from build123d import *

# Parameters (mm, degrees)
F0_R        = 8.4621636151
F0_R_2      = 8.6410874337
F1_DEPTH    = 50
F4_T1_DEPTH = 125
F4_T3_DEPTH = 75.1791274175
F4_T8_DEPTH = 127.0995380357


# Not quite as in the source:
# - a fillet or chamfer that OpenCascade refuses, or shapes differently, is made with other operations: its cross-section is extruded or revolved along the edge and cut away or added
# - a feature of the source that left no trace in its solid (it failed there, or was rolled back) is left out


with BuildPart() as f1:
    # F0 (on Front) → F1 (new body)
    with BuildSketch(Plane.XZ):
        with BuildLine():
            Line((-12.9085844383, 52.6810027659), (-60.1237900555, 52.6810027659))
            Line((-60.1237900555, 52.6810027659), (-60.1237900555, 27.209569862))
            ThreePointArc((-60.1237900555, 27.209569862), (-40.7058920955, 7.7916719019), (-60.1237900555, -11.6262260581))
            Line((-60.1237900555, -11.6262260581), (-60.1237900555, -42.4471646547))
            Line((-60.1237900555, -42.4471646547), (-12.2108235955, -42.4471646547))
            Line((-12.2108235955, -42.4471646547), (-12.2108235955, -22.2120806575))
            Line((-12.2108235955, -22.2120806575), (11.7456596345, -22.2120806575))
            Line((11.7456596345, -22.2120806575), (11.7456596345, -42.4471646547))
            Line((11.7456596345, -42.4471646547), (60.588978231, -42.4471646547))
            Line((60.588978231, -42.4471646547), (60.588978231, 0))
            Line((60.588978231, 0), (13.5322010265, 0))
            ThreePointArc((13.5322010265, 0), (4.0349011674, 7.5009376742), (13.5322010265, 15.0018753484))
            Line((13.5322010265, 15.0018753484), (60.588978231, 15.0018753484))
            Line((60.588978231, 15.0018753484), (60.588978231, 52.6810027659))
            Line((60.588978231, 52.6810027659), (8.4894401953, 52.6810027659))
            Line((8.4894401953, 52.6810027659), (8.4894401953, 30.5852182209))
            Line((8.4894401953, 30.5852182209), (-12.9085844383, 30.5852182209))
            Line((-12.9085844383, 30.5852182209), (-12.9085844383, 52.6810027659))
        make_face()
        with Locations((40.4487065971, -18.1611850858)):
            Circle(F0_R, mode=Mode.SUBTRACT)
        with Locations((37.1295772493, 35.4981198907)):
            Circle(F0_R_2, mode=Mode.SUBTRACT)
    extrude(amount=F1_DEPTH)

    # F4: fillet of radius 15 on 3 edges, made by hand

    # F4_s2 → F4_t1 (cut)
    with BuildSketch(Plane.XZ.offset(-37.5)):
        with BuildLine():
            ThreePointArc((45.588978231, -42.4471646547), (56.1955799488, -38.0537663725), (60.588978231, -27.4471646547))
            Line((60.588978231, -27.4471646547), (60.588978231, -42.4471646547))
            Line((60.588978231, -42.4471646547), (45.588978231, -42.4471646547))
        make_face()
    extrude(amount=F4_T1_DEPTH, mode=Mode.SUBTRACT)

    # F4_s4 → F4_t3 (cut)
    with BuildSketch(Plane.XY.offset(15.0018753484)):
        with BuildLine():
            ThreePointArc((60.588978231, -15), (56.1955799488, -4.3933982822), (45.588978231, 0))
            Line((45.588978231, 0), (60.588978231, 0))
            Line((60.588978231, 0), (60.588978231, -15))
        make_face()
    extrude(amount=F4_T3_DEPTH, mode=Mode.SUBTRACT)


with BuildPart() as f4_tool6:
    # F4_s7 → F4_t8 (new body)
    with BuildSketch(Plane.YZ.offset(98.088978231)):
        with BuildLine():
            ThreePointArc((-35, 52.6810027659), (-45.6066017178, 48.2876044837), (-50, 37.6810027659))
            Line((-50, 37.6810027659), (-50, 52.6810027659))
            Line((-50, 52.6810027659), (-35, 52.6810027659))
        make_face()
    extrude(amount=-F4_T8_DEPTH)

    split(bisect_by=Plane.YZ.offset(-12.9085844383), keep=Keep.TOP)


with BuildPart() as f1_1:
    add(f1.part)

    # F4_t5: cut F4_tool6
    add(f4_tool6.part, mode=Mode.SUBTRACT)


solid = f1_1.part
Model file for the job. Use its own axes, mm. A direction names the side the tool comes from. Round coordinates to 2 decimals unless told otherwise and drop trailing zeros. Loops run counter-clockwise (first coordinate to the right, second up) from the corner with the lowest first, then second, coordinate; pieces in that order, holes last.
1. Band-saw the part on D-D, the plane z = -24.5. List the corners of the cut face in (x, y).
Check values:
outline: (-60.12, -50) - (-12.21, -50) - (-12.21, 0) - (-60.12, 0) - close; (11.75, -50) - (34.84, -50) - (34.84, 0) - (11.75, 0) - close; (46.05, -50) - (60.59, -50) - (60.59, 0) - (46.05, 0) - close
2. Wall check: probe 1 along X at (y, z) = (-12, 37); probe 2 along Z at (x, y) = (45, -12); probe 3 along Z at (x, y) = (4, -32.5). Give the ranges that are in metal, low to high.
Check values:
probe 1: x = -60.12 to -12.91, 8.49 to 28.62, 45.64 to 60.29
probe 2: z = -42.45 to -25.3, -11.03 to 0, 15 to 31.93, 39.07 to 52.68
probe 3: z = -22.21 to 30.59
3. Mould opens along Z. For faces 5 (the flat face through (28, -25, -42.447)), 6 (the flat face through (37, -25, 15.002)), 7 (the flat face through (60.589, -25, -14)) say: +Z half, -Z half, draft (parallel to the pull), parting line (faces both ways), or undercut.
Check values:
face 5: -Z half
face 6: undercut
face 7: draft
4. Band-saw the part on A-A, the plane x = -43. List the corners of the cut face in (y, z).
Check values:
outline: (-50, -42.45) - (0, -42.45) - (0, -1.36) - (-50, -1.36) - close; (-50, 16.95) - (0, 16.95) - (0, 52.68) - (-50, 52.68) - close
5. Tool access for faces 1 (the cylindrical face through (56.3, -4.5, 33.6)), 2 (the flat face through (-12.909, -25, 41)), 3 (the cylindrical face through (34.904, -45.489, 48.404)), 4 (the flat face through (37, -25, 0)): list every direction of +Z, -Z, +X, -X, +Y, -Y with a clear straight run to the whole face (end or side of a thin tool).
Check values:
face 1: +Z, +X, +Y
face 2: +Z, +Y, -Y
face 3: +Z, +X, -Y
face 4: +X, +Y, -Y
6. Band-saw the part on C-C, the plane y = -39.5. List the corners of the cut face in (x, z), and give its area (3 significant figures).
Check values:
outline: (-60.12, -42.45) - (-12.21, -42.45) - (-12.21, -22.21) - (11.75, -22.21) - (11.75, -42.45) - (45.59, -42.45) arc R15 ccw to (60.59, -27.45) - (60.59, 0) - (13.53, 0) arc R7.71 cw (long way) to (13.53, 15) - (60.59, 15) - (60.59, 51.99) - (8.49, 51.99) - (8.49, 30.59) - (-12.91, 30.59) - (-12.91, 52.68) - (-60.12, 52.68) - (-60.12, 27.21) arc R19.42 cw to (-60.12, -11.63) - close; hole circle Ø17.28 at (37.13, 35.5); hole circle Ø16.92 at (40.45, -18.16)
area: 8,560 mm2
7. Band-saw the part on B-B, the plane z = 47.5. List the corners of the cut face in (x, y), and give its area (3 significant figures).
Check values:
outline: (-60.12, -50) - (-12.91, -50) - (-12.91, 0) - (-60.12, 0) - close; (8.49, -46.34) - (60.59, -46.34) - (60.59, -15) arc R15 ccw to (45.59, 0) - (8.49, 0) - close
area: 4,730 mm2
8. Drop a flat-ended pin along its axis: P1, Ø17, axis at x = -1, y = -24, coming from the +Z side. Give the stop position or say it passes through.
Check values:
P1: stops at z = 30.59
